from build123d import *

# Parameters (mm, degrees)
CROQUIS1_R                 = 3.05
CROQUIS1_R_2               = 1.5
SALIENTE_EXTRUIR1_DEPTH    = 11.8
TALADRO_ROSCADO_M51_D      = 4.2
CROQUIS2_W                 = 10.5
CROQUIS2_H                 = 4.3
CORTAR_EXTRUIR1_DEPTH      = 18
CORTAR_EXTRUIR6_DEPTH      = 58.488085722
CORTAR_EXTRUIR6_DEPTH_BACK = 58.488085722
CROQUIS13_R                = 2.5
CROQUIS27_R                = 3.1
CORTAR_EXTRUIR8_DEPTH      = 10
CROQUIS31_R                = 3.75
CORTAR_EXTRUIR9_DEPTH      = 5
CORTAR_EXTRUIR12_DEPTH     = 59.884038604
CHAFL_N2_SIZE              = 4
CHAFL_N3_SIZE              = 2
CORTAR_EXTRUIR17_DEPTH     = 62.212172011
CROQUIS46_W                = 28.049554897
CROQUIS46_H                = 7
CORTAR_EXTRUIR18_DEPTH     = 59.884038604
TALADRO_ROSCADO_M31_D      = 2.5
TALADRO_ROSCADO_M31_DEPTH  = 8.5
REDONDEO2_R                = 0.75
CHAFL_N5_SIZE              = 0.6
CHAFL_N5_SIZE2             = 1.039230485
CHAFL_N6_SIZE              = 4


with BuildPart() as part:
    # Croquis1 → Saliente-Extruir1 (new body)
    with BuildSketch(Plane(origin=(0, 0, 0), x_dir=(1, 0, 0), z_dir=(0, 1, 0))):
        with BuildLine():
            Line((16.9, -8.95), (15.65, -8.95))
            ThreePointArc((15.65, -8.95), (12.702454225, -9.911191525), (10.888170856, -12.425210439))
            Line((10.888170856, -12.425210439), (9.423737687, -16.998550083))
            ThreePointArc((9.423737687, -16.998550083), (7.700168487, -19.386868052), (4.9, -20.3))
            Line((4.9, -20.3), (-6, -20.3))
            Line((-6, -20.3), (-6, 6))
            Line((-6, 6), (54, 6))
            Line((54, 6), (54, -15.5))
            Line((54, -15.5), (21.9, -15.5))
            Line((21.9, -15.5), (21.9, -13.95))
            ThreePointArc((21.9, -13.95), (20.435533906, -10.414466094), (16.9, -8.95))
        make_face()
        with Locations(Location((0, 0, 0), (0, 0, 270))):
            Circle(CROQUIS1_R, mode=Mode.SUBTRACT)
        with Locations(Location((4.9, -15.55, 0), (0, 0, 270))):
            Circle(CROQUIS1_R_2, mode=Mode.SUBTRACT)
    extrude(amount=SALIENTE_EXTRUIR1_DEPTH)

    # Taladro roscado M51 (through all)
    with Locations(Plane(origin=(0, 11.8, 0), x_dir=(1, 0, 0), z_dir=(0, 1, 0))):
        with Locations((4.9, -15.55)):
            Hole(TALADRO_ROSCADO_M51_D / 2)

    # Croquis2 → Cortar-Extruir1 (cut)
    with BuildSketch(Plane.ZY.offset(6)):
        with Locations((15.05, 5.9)):
            Rectangle(CROQUIS2_W, CROQUIS2_H)
    extrude(amount=-CORTAR_EXTRUIR1_DEPTH, mode=Mode.SUBTRACT)

    # Croquis13 → Cortar-Extruir6 (cut, two sides: drawn at the far end of the back side and taken through both)
    with BuildSketch(Plane.XY.offset(9.8).offset(-CORTAR_EXTRUIR6_DEPTH_BACK)):
        with Locations((10.8, 5.9)):
            Circle(CROQUIS13_R)
    extrude(amount=CORTAR_EXTRUIR6_DEPTH + CORTAR_EXTRUIR6_DEPTH_BACK, mode=Mode.SUBTRACT)

    # Croquis27 → Cortar-Extruir8 (cut)
    with BuildSketch(Plane(origin=(0, 0, -6), x_dir=(-1, 0, 0), z_dir=(0, 0, -1))):
        with Locations((-10.8, 5.9)):
            Circle(CROQUIS27_R)
    extrude(amount=-CORTAR_EXTRUIR8_DEPTH, mode=Mode.SUBTRACT)

    # Croquis31 → Cortar-Extruir9 (cut)
    with BuildSketch(Plane.XY.offset(15.5)):
        with Locations((37.5, 5.9)):
            Circle(CROQUIS31_R)
    extrude(amount=-CORTAR_EXTRUIR9_DEPTH, mode=Mode.SUBTRACT)

    # Croquis34 → Cortar-Extruir12 (cut, through all)
    with BuildSketch(Plane.XZ):
        with BuildLine():
            Line((54, 6.5), (41, 6.5))
            ThreePointArc((41, 6.5), (29.819660113, 3.083123952), (22.459503782, -6))
            Line((22.459503782, -6), (54, -6))
            Line((54, -6), (54, 6.5))
        make_face()
    extrude(amount=-CORTAR_EXTRUIR12_DEPTH, mode=Mode.SUBTRACT)

    # Chafl_n2
    chafl_n2_edges = [part.edges().sort_by_distance(p)[0] for p in [
        (-6, 5.9, -6),
    ]]
    chamfer(chafl_n2_edges, length=CHAFL_N2_SIZE)

    # Chafl_n3
    chafl_n3_edges = [part.edges().sort_by_distance(p)[0] for p in [
        (54, 5.9, 6.5),
    ]]
    chamfer(chafl_n3_edges, length=CHAFL_N3_SIZE)

    # Croquis35 → Cortar-Revoluci_n1 (revolve, cut)
    with BuildSketch(Plane(origin=(0, 5.9, 0), x_dir=(-1, 0, 0), z_dir=(0, -1, 0)), mode=Mode.PRIVATE) as cortar_revoluci_n1_sk:
        Polygon((-13.9, -4), (-10.8, -9.369357503), (-10.8, -4), align=None)
    revolve(cortar_revoluci_n1_sk.sketch.rotate(Axis((10.8, 5.9, 4), (0, 0, -1)), 87.978853678), axis=Axis((10.8, 5.9, 4), (0, 0, -1)), mode=Mode.SUBTRACT)

    # Croquis45 → Cortar-Extruir17 (cut, through all)
    with BuildSketch(Plane(origin=(0, 0, -6), x_dir=(-1, 0, 0), z_dir=(0, 0, -1))):
        with BuildLine():
            Line((-22.3, 2.4), (-28.3, 2.4))
            ThreePointArc((-28.3, 2.4), (-31.8, 5.9), (-28.3, 9.4))
            Line((-28.3, 9.4), (-22.3, 9.4))
            ThreePointArc((-22.3, 9.4), (-18.8, 5.9), (-22.3, 2.4))
        make_face()
    extrude(amount=-CORTAR_EXTRUIR17_DEPTH, mode=Mode.SUBTRACT)

    # Croquis46 → Cortar-Extruir18 (cut, through all)
    with BuildSketch(Plane.XZ):
        with Locations((18.774777449, -2.5)):
            Rectangle(CROQUIS46_W, CROQUIS46_H)
    extrude(amount=-CORTAR_EXTRUIR18_DEPTH, mode=Mode.SUBTRACT)

    # Taladro roscado M31
    with Locations(Plane(origin=(0, 0, 1), x_dir=(-1, 0, 0), z_dir=(0, 0, -1))):
        with Locations((-17.8, 2.3)):
            Hole(TALADRO_ROSCADO_M31_D / 2, depth=TALADRO_ROSCADO_M31_DEPTH)

    # Redondeo2
    redondeo2_edges = [part.edges().sort_by_distance(p)[0] for p in [
        (4.75, 5.9, 1),
    ]]
    fillet(redondeo2_edges, radius=REDONDEO2_R)

    # Chafl_n5
    chafl_n5_edges = [part.edges().sort_by_distance(p)[0] for p in [
        (13.9, 5.9, 1),
    ]]
    chafl_n5_side = [part.faces().sort_by_distance(p)[0] for p in [
        (15.082931418, 6.005477059, 1),
    ]]
    chamfer(chafl_n5_edges, length=CHAFL_N5_SIZE, length2=CHAFL_N5_SIZE2, reference=chafl_n5_side[0])

    # Chafl_n6
    chafl_n6_edges = [part.edges().sort_by_distance(p)[0] for p in [
        (-6, 9.925, 20.3),
        (-6, 1.875, 20.3),
    ]]
    chamfer(chafl_n6_edges, length=CHAFL_N6_SIZE)


solid = part.part
Here's how the part is built. I have some questions about the finished solid (model axes, mm). A direction names the side the tool comes from. Round coordinates to 2 decimals unless told otherwise and drop trailing zeros. Loops run counter-clockwise (first coordinate to the right, second up) from the corner with the lowest first, then second, coordinate; pieces in that order, holes last.
1. If we section it at B-B on y = 7.25: Count the separate pieces of the cut face and the enclosed holes in it, plus the area to 3 significant figures.
Answer list:
separate pieces: 3
enclosed holes: 1
area: 385 mm2
2. If I drill on line 1 along Y through (x, z) = (10.8, 3.6); line 2 along Y through (x, z) = (37.5, 12.4); line 3 along X through (y, z) = (7.5, 7), over which ranges is the centre line in solid material (lowest first)?
Answer list:
line 1: y = 0 to 2.8, 9 to 11.8
line 2: y = 0 to 2.15, 9.65 to 11.8
line 3: x = -6 to 8.88, 12.72 to 19.19, 31.41 to 52.5
3. We'd pull the mould along X, two halves only. Please class faces 1 (the face through (2, 6, 9.8)), 2 (the face through (18.247, 5.817, 9.135)), 3 (the face through (53, 5.8, 7.5)): +X half, -X half, draft (parallel to the pull), parting line (faces both ways), or undercut.
Answer list:
face 1: draft
face 2: undercut
face 3: +X half
4. Which directions (+Z, -Z, +X, -X, +Y, -Y) give clear straight access to the entire face, cutting with the end or side of a thin tool? Please do faces 4 (the face through (9.13, 8.51, 3.01)), 5 (the face through (2, 8.05, 15)), 6 (the face through (4.75, 6, -3)), 7 (the face through (21.9, 1, 15)), 8 (the face through (18.8, 6, 4.9)).
Answer list:
face 4: -Z
face 5: +Z, -X
face 6: -Z, +X, +Y, -Y
face 7: +Z, +Y, -Y
face 8: +Z, -Z
5. If we section it at C-C on x = 49.5: Write out the boundary of the cut face in (y, z), plus the area to 3 significant figures.
Answer list:
outline: (0, 6.5) - (11.8, 6.5) - (11.8, 15.5) - (0, 15.5) - close
area: 106 mm2
6. For P1, Ø2.5, axis at x = 4.9, z = 15.55, coming from the -Y side; P2, Ø11.5, axis at x = 4.5, z = 12.5, coming from the -Y side; P3, Ø3, axis at x = 42, y = 4.5, coming from the -Z side, each with a flat end and sliding along its axis, tell me the tip position at first contact or that it passes through.
Answer list:
P1: passes through
P2: stops at y = 0
P3: stops at z = 6.49
7. If we section it at A-A on x = 37.5: Write out the boundary of the cut face in (y, z).
Answer list:
outline: (0, 6.19) - (11.8, 6.19) - (11.8, 15.5) - (9.65, 15.5) - (9.65, 10.5) - (2.15, 10.5) - (2.15, 15.5) - (0, 15.5) - close
